The model under review builds one solid part; all positions refer to its coordinate system, in mm. Round coordinates to 2 decimals unless told otherwise and drop trailing zeros. Order: outer loops, then holes, each group sorted by start corner. A loop starts at its lowest first (then second) coordinate and runs counter-clockwise, first axis right, second up. Notation, with made-up numbers: (84.5, -7.75) - (106.5, -7.75) arc R4 cw to (106.5, -1.75) - close; hole circle Ø9 at (75.5, 74). An arc over 180 degrees is marked (long way). One line per question, with ' | ' between items. Start each with the question number.
Item 1: For L1, parallel to Y at x = 2, z = 0.95; L2, parallel to Y at x = 0, z = 1.1; L3, parallel to Y at x = -2.5, z = 0.9, list the stretches that pass through material, from the lowest coordinate up. Write a range as [from, to].
Item 2: Add section B-B on y = -3.75. State the section outline as (x, z) points (3 decimals), and give its area (3 significant figures).
Item 3: Add section D-D on x = 0. State the section outline as (y, z) points (3 decimals).
Item 4: Add section C-C on z = 1. State the section outline as (x, y) points (3 decimals), and give its area (3 significant figures).
Item 5: Insertion check: pin 1 Ø5 at (x, y) = (3.5, 1) entering from +Z. The pin has a flat end and moves straight along its axis. Give the tip position at first contact, or say it passes through.
Item 6: Add section A-A on x = -3.5. State the section outline as (y, z) points (3 decimals), and give its area (3 significant figures).
from build123d import *

# Parameters (mm, degrees)
SKETCH1_R                 = 7.9
EXTRUDE1_DEPTH            = 0.775
SKETCH34_R                = 0.5
F_056_250_SNAP_RING_DEPTH = 0.775
SKETCH35_R                = 7.9
CUT_EXTRUDE1_DEPTH        = 0.775


with BuildPart() as part:
    # Sketch1 → Extrude1 (new body)
    with BuildSketch(Plane.XY):
        with Locations(Location((0, 0, 0), (0, 0, 180))):
            Circle(SKETCH1_R)
    extrude(amount=EXTRUDE1_DEPTH)

    # Sketch34 → 056-250 Snap Ring (add)
    with BuildSketch(Plane.XY.offset(0.775)):
        with BuildLine():
            Line((-1.357948468, -6.654737152), (-1.740532253, -7.705877463))
            ThreePointArc((-1.740532253, -7.705877463), (0, 7.9), (1.740532253, -7.705877463))
            Line((1.740532253, -7.705877463), (1.357948468, -6.654737152))
            ThreePointArc((1.357948468, -6.654737152), (1.863757747, -5.411747949), (3.15093243, -5.791282558))
            ThreePointArc((3.15093243, -5.791282558), (3.849974822, -6.257880122), (4.657974592, -6.026558003))
            ThreePointArc((4.657974592, -6.026558003), (0, 6.49), (-4.657974592, -6.026558003))
            ThreePointArc((-4.657974592, -6.026558003), (-3.849974822, -6.257880122), (-3.15093243, -5.791282558))
            ThreePointArc((-3.15093243, -5.791282558), (-1.863757747, -5.411747949), (-1.357948468, -6.654737152))
        make_face()
        with Locations((2.297641088, -6.312717009)):
            Circle(SKETCH34_R, mode=Mode.SUBTRACT)
        with Locations((-2.297641088, -6.312717009)):
            Circle(SKETCH34_R, mode=Mode.SUBTRACT)
    extrude(amount=F_056_250_SNAP_RING_DEPTH)

    # Sketch35 → Cut-Extrude1 (cut)
    with BuildSketch(Plane(origin=(0, 0, 0), x_dir=(-1, 0, 0), z_dir=(0, 0, -1))):
        Circle(SKETCH35_R)
    extrude(amount=-CUT_EXTRUDE1_DEPTH, mode=Mode.SUBTRACT)


solid = part.part
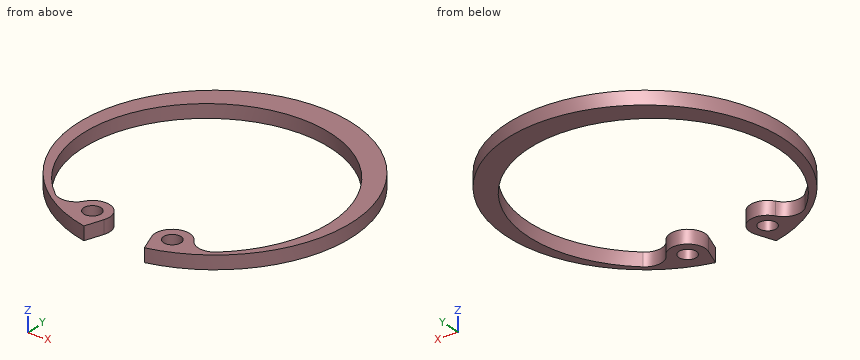
Determined:
1) L1: [-7.64, -6.71], [-5.91, -5.36], [6.2, 7.64] | L2: [6.49, 7.9] | L3: [-7.49, -6.77], [-5.86, -5.33], [6.04, 7.49]
2) outline: (-6.953, 0.775) - (-6.408, 0.775) - (-6.408, 1.55) - (-6.953, 1.55) - close; (6.408, 0.775) - (6.953, 0.775) - (6.953, 1.55) - (6.408, 1.55) - close | area: 0.845 mm2
3) outline: (6.49, 0.775) - (7.9, 0.775) - (7.9, 1.55) - (6.49, 1.55) - close
4) outline: (-4.658, -6.027) arc R7.125 cw (long way) to (4.658, -6.027) arc R1 cw to (3.151, -5.791) arc R1 ccw to (1.358, -6.655) - (1.741, -7.706) arc R7.9 ccw (long way) to (-1.741, -7.706) - (-1.358, -6.655) arc R1 ccw to (-3.151, -5.791) arc R1 cw to start; hole circle Ø1 at (-2.298, -6.313); hole circle Ø1 at (2.298, -6.313) | area: 42.3 mm2
5) pin 1: through
6) outline: (-7.082, 0.775) - (-6.133, 0.775) - (-6.133, 1.55) - (-7.082, 1.55) - close; (5.571, 0.775) - (7.082, 0.775) - (7.082, 1.55) - (5.571, 1.55) - close | area: 1.91 mm2
